The listing builds one solid part. Answer for the finished solid, in the listing's coordinates (mm). Face numbers are marked on the shaded views. A direction names the side the tool comes from. Coordinates: 2 decimals unless noted, no trailing zeros. Write each loop counter-clockwise with the first axis right and the second up, starting at its lowest first coordinate (ties: lowest second). Pieces come first, ordered by that corner, then holes.
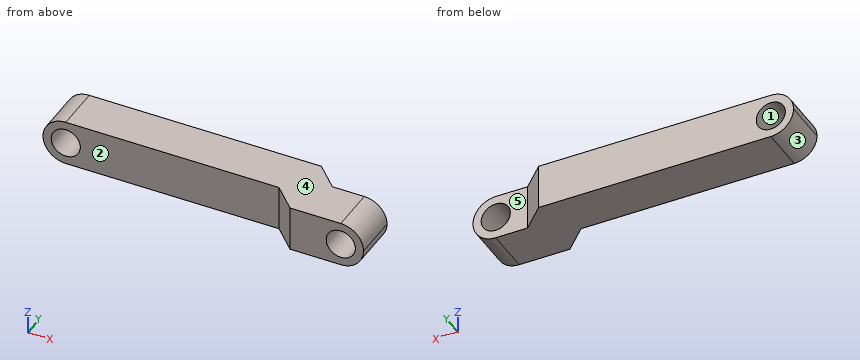
```python
from build123d import *

# Parameters (mm, degrees)
F1_DEPTH = 7.9375
F2_R     = 3.96874
F3_R     = 2.54
F4_DEPTH = 11.90625


# Not quite as in the source:
# - a fillet or chamfer is up to 0.001 mm smaller than in the source, because OpenCascade refuses the exact size


with BuildPart() as f1:
    # F0 (on Top) → F1 (new body)
    with BuildSketch(Plane.XY):
        Polygon((44.45, 0), (0, 0), (0, -7.9375), (41.1621798487, -7.9375), (45.1309298487, -11.90625), (57.94375, -11.90625), (57.94375, -3.96875), (48.41875, -3.96875), align=None)
    extrude(amount=F1_DEPTH)

    # F2 (radius 3.96875 in the source; OpenCascade refuses exactly that, so slightly less here)
    f2_edges = [f1.edges().sort_by_distance(p)[0] for p in [
        (0, -3.96875, 0),
        (0, -3.96875, 7.9375),
        (57.94375, -7.9375, 0),
        (57.94375, -7.9375, 7.9375),
    ]]
    fillet(f2_edges, radius=F2_R)

    # F3 (on face) → F4 (cut, through all)
    with BuildSketch(Plane(origin=(0, 0, 0), x_dir=(-1, 0, 0), z_dir=(0, 1, 0))):
        with Locations((-3.96875, 3.96875)):
            Circle(F3_R)
        with Locations((-53.975, 3.96875)):
            Circle(F3_R)
    extrude(amount=-F4_DEPTH, mode=Mode.SUBTRACT)


solid = f1.part
```
(1) For a pull along Z with two mould halves and no side action, classify the marked faces 1, 2 and 3 as pulls with the +Z half, pulls with the -Z half, needs draft (parallel to the pull), parting line crosses it, or undercut.
(2) Which of the six approach directions +Z, -Z, +X, -X, +Y, -Y give full straight-line access (tool end or side, diameter ignored) to the marked faces 4 and 5?
(3) This flat-tipped pin is pushed along its axis until it touches: pin 1 (2 mm diameter, centred on y = -9, z = 6, fed in from -X). Where does it stop, or does it pass through?
(4) Section B-B, the plane z = 2.5 is taken. Write down the section's boundary in (x, y), plus the area to 3 significant figures.
(5) Section C-C, the plane y = -7.25 is taken. State how many separate pieces and enclosed holes the cut face has, plus the area to 3 significant figures.
(6) Section D-D, the plane x = 28 is taken. Write down the section's boundary in (y, z), plus the area to 3 significant figures.
(7) Find the intervals of material crossed by probe 1 along X at (y, z) = (-4, 4); probe 2 along X at (y, z) = (-6.25, 4.25); probe 3 along Y at (x, z) = (25, 5.5), in increasing order.
Solution:
1. face 1: undercut
1. face 2: needs draft
1. face 3: pulls with the -Z half
2. face 4: +Z, +X, -X, +Y, -Y
2. face 5: +Z, -Z, +X, +Y
3. pin 1: stops at x = 41.22
4. outline: (0.28, -7.94) - (1.9, -7.94) - (1.9, 0) - (0.28, 0) - close; (6.04, -7.94) - (41.16, -7.94) - (45.13, -11.91) - (51.9, -11.91) - (51.9, -3.97) - (48.42, -3.97) - (44.45, 0) - (6.04, 0) - close; (56.05, -11.91) - (57.66, -11.91) - (57.66, -3.97) - (56.05, -3.97) - close
4. area: 403 mm2
5. separate pieces: 1
5. enclosed holes: 2
5. area: 406 mm2
6. outline: (-7.94, 0) - (0, 0) - (0, 7.94) - (-7.94, 7.94) - close
6. area: 63.0 mm2
7. probe 1: x = 0 to 1.43, 6.51 to 51.44, 56.51 to 57.94
7. probe 2: x = 0.01 to 1.44, 6.49 to 51.45, 56.5 to 57.93
7. probe 3: y = -7.94 to 0
